Geometry check sheet. Reference: the model listing, model coordinates, mm. Round coordinates to 2 decimals unless told otherwise and drop trailing zeros. Write each loop counter-clockwise with the first axis right and the second up, starting at its lowest first coordinate (ties: lowest second). Pieces come first, ordered by that corner, then holes. Notation, with made-up numbers: M -33,-1 L -4,-1 A29 cw -4,35 Z; hole C 63.5,30.5 d1. An arc over 180 degrees is marked long. One line per item, written item: value. Start each with the question number.
1. Section check D-D (x = 18). Record the boundary of the cut face in (y, z), and give its area (3 significant figures).
2. Section check C-C (x = -18). Record the boundary of the cut face in (y, z).
3. Section check A-A (z = 2.25). Record the boundary of the cut face in (x, y).
4. Release check for a two-part mould opening along Y. For faces 1 (the flat face through (20, -10, 0)), 2 (the cylindrical face through (-16.38, -10.51, 3.63)), 3 (the flat face through (0, 0, 12)) record: pulls with the +Y half, pulls with the -Y half, needs draft (parallel to the pull), parting line crosses it, or undercut.
5. Scan lines: probe 1 along Y at (x, z) = (-18, 5); probe 2 along X at (y, z) = (-15, 9.75); probe 3 along X at (y, z) = (-14.5, 3.25). Record each from-to range of solid material in increasing order. Write a range as [from, to].
6. Depth check by flat-ended pin: P1, Ø5, axis at x = -15, y = -16.5, coming from the +Z side; P2, Ø1, axis at x = -1.5, y = -17.5, coming from the +Z side; P3, Ø8, axis at y = -5.5, z = 15, coming from the -X side. Enter the tip coordinate at first touch or a pass-through.
7. Section check B-B (y = -10). Record the boundary of the cut face in (x, z).
from build123d import *

# Parameters (mm, degrees)
F1_DEPTH = 20
F2_R     = 1.7
F3_R     = 1.75
F4_DEPTH = 17.001


with BuildPart() as f1:
    # F0 (on Front) → F1 (new body)
    with BuildSketch(Plane.XZ):
        with BuildLine():
            ThreePointArc((-15, 0), (0, 11), (15, 0))
            Line((15, 0), (21, 0))
            ThreePointArc((21, 0), (0, 17), (-21, 0))
            Line((-21, 0), (-15, 0))
        make_face()
    extrude(amount=F1_DEPTH)

    # F2 (on face) + F3 (on face) → F4 (cut, through all)
    with BuildSketch(Plane(origin=(0, 0, 0), x_dir=(1, 0, 0), z_dir=(0, 0, -1))):
        with Locations((-18, 10)):
            Circle(F2_R)
    with BuildSketch(Plane(origin=(0, 0, 0), x_dir=(1, 0, 0), z_dir=(0, 0, -1))):
        with Locations((18, 10)):
            Circle(F3_R)
    extrude(amount=-F4_DEPTH, mode=Mode.SUBTRACT)


solid = f1.part
Result sheet:
1. outline: M -20,0 L -11.75,0 L -11.75,7.23 L -20,7.23 Z; M -8.25,0 L 0,0 L 0,7.23 L -8.25,7.23 Z
1. area: 119 mm2
2. outline: M -20,0 L -11.7,0 L -11.7,7.23 L -20,7.23 Z; M -8.3,0 L 0,0 L 0,7.23 L -8.3,7.23 Z
3. outline: M -20.39,-20 L -14.09,-20 L -14.09,0 L -20.39,0 Z; M 14.09,-20 L 20.39,-20 L 20.39,0 L 14.09,0 Z; hole C -18,-10 d3.4; hole C 18,-10 d3.5
4. face 1: needs draft
4. face 2: undercut
4. face 3: pulls with the +Y half
5. probe 1: y = [-20, -11.7], [-8.3, 0]
5. probe 2: x = [-16.09, -6.14], [6.14, 16.09]
5. probe 3: x = [-20.03, -13.55], [13.55, 20.03]
6. P1: stops at z = 12.99
6. P2: stops at z = 16.98
6. P3: stops at x = -14.89
7. outline: M -21,0 L -19.7,0 L -19.7,4.07 A21.47 ccw Z; M -16.3,0 L -15,0 A15.73 cw 15,0 L 16.25,0 L 16.25,9.56 A21.47 ccw -16.3,9.5 Z; M 19.75,0 L 21,0 A21.47 ccw 19.75,3.95 Z
